from build123d import *
from OCP.BRepFilletAPI import BRepFilletAPI_MakeChamfer

# Parameters (mm, degrees)
SKETCH1_W           = 50
SKETCH1_H           = 40
BODY_DEPTH          = 12
FILLETBODY_R        = 3
SKETCH3_R           = 3.75
BOLT_EXTRUDE_DEPTH  = 1
BOLT_DEPTH          = 10
BOLT_DEPTH_BACK     = 16
SKETCH4_R           = 1.5
SKETCH41_R          = 1.575
CHANNEL1_DEPTH      = 57
SKETCH42_R          = 2.575
INLET_DEPTH         = 5
OUTLET_START        = -5
SKETCH43_R          = 2.575
OUTLET_DEPTH        = 5
SKETCH44_R          = 15
WINDOW_DEPTH        = 5.5
SKETCH45_W          = 16
SKETCH45_H          = 10
FLOWCH_DEPTH        = 5.575
SKETCH46_W          = 10
SKETCH46_H          = 10
WINDOW_HOLE_DEPTH   = 16
SKETCH49_R          = 1.5
FIXHOLES_DEPTH      = 2
GASKET_DEPTH        = 1
CHAMFER_FLOW_SIZE   = 0.5
CHAMFER_FLOW_SIZE_2 = 3


with BuildPart() as part:
    # Sketch1 → Body (new body)
    with BuildSketch(Plane(origin=(0, 0, 0), x_dir=(1, 0, 0), z_dir=(0, 1, 0))):
        Rectangle(SKETCH1_W, SKETCH1_H)
    extrude(amount=BODY_DEPTH)

    # FilletBody
    filletbody_edges = [part.edges().sort_by_distance(p)[0] for p in [
        (-25, 6, -20),
        (25, 6, -20),
        (25, 6, 20),
        (-25, 6, 20),
    ]]
    fillet(filletbody_edges, radius=FILLETBODY_R)

    # Sketch3 → Bolt extrude (add)
    with BuildSketch(Plane(origin=(0, 12, 0), x_dir=(1, 0, 0), z_dir=(0, 1, 0))):
        with Locations(Location((-17.5, 12.5, 0), (0, 0, 270))):
            Circle(SKETCH3_R)
        with Locations(Location((17.5, 12.5, 0), (0, 0, 90))):
            Circle(SKETCH3_R)
        with Locations(Location((17.5, -12.5, 0), (0, 0, 270))):
            Circle(SKETCH3_R)
        with Locations(Location((-17.5, -12.5, 0), (0, 0, 90))):
            Circle(SKETCH3_R)
    extrude(amount=BOLT_EXTRUDE_DEPTH)

    # Sketch4 → Bolt (cut, two sides: drawn at the far end of the back side and taken through both)
    with BuildSketch(Plane(origin=(0, 13, 0), x_dir=(1, 0, 0), z_dir=(0, 1, 0)).offset(-BOLT_DEPTH_BACK)):
        with Locations(Location((-17.5, 12.5, 0), (0, 0, 270))):
            Circle(SKETCH4_R)
        with Locations(Location((17.5, 12.5, 0), (0, 0, 90))):
            Circle(SKETCH4_R)
        with Locations(Location((17.5, -12.5, 0), (0, 0, 270))):
            Circle(SKETCH4_R)
        with Locations(Location((-17.5, -12.5, 0), (0, 0, 90))):
            Circle(SKETCH4_R)
    extrude(amount=BOLT_DEPTH + BOLT_DEPTH_BACK, mode=Mode.SUBTRACT)

    # Sketch41 → Channel1 (cut)
    with BuildSketch(Plane.ZY.offset(25)):
        with Locations((0, 4)):
            Circle(SKETCH41_R)
    extrude(amount=-CHANNEL1_DEPTH, mode=Mode.SUBTRACT)

    # Sketch42 → Inlet (cut)
    with BuildSketch(Plane.ZY.offset(25)):
        with Locations((0, 4)):
            Circle(SKETCH42_R)
    extrude(amount=-INLET_DEPTH, mode=Mode.SUBTRACT)

    # Sketch43 → Outlet (cut)
    with BuildSketch(Plane(origin=(25, 0, 0), x_dir=(0, 0, -1), z_dir=(1, 0, 0)).offset(OUTLET_START)):
        with Locations(Location((0, 4, 0), (0, 0, 180))):
            Circle(SKETCH43_R)
    extrude(amount=OUTLET_DEPTH, mode=Mode.SUBTRACT)

    # Sketch44 → Window (cut)
    with BuildSketch(Plane(origin=(0, 12, 0), x_dir=(1, 0, 0), z_dir=(0, 1, 0))):
        with Locations(Location((0, 0, 0), (0, 0, 270))):
            Circle(SKETCH44_R)
    extrude(amount=-WINDOW_DEPTH, mode=Mode.SUBTRACT)

    # Sketch45 → FlowCh (cut)
    with BuildSketch(Plane.XZ):
        Rectangle(SKETCH45_W, SKETCH45_H)
    extrude(amount=-FLOWCH_DEPTH, mode=Mode.SUBTRACT)

    # Sketch46 → Window_hole (cut)
    with BuildSketch(Plane(origin=(0, 6.5, 0), x_dir=(1, 0, 0), z_dir=(0, 1, 0))):
        Rectangle(SKETCH46_W, SKETCH46_H)
    extrude(amount=-WINDOW_HOLE_DEPTH, mode=Mode.SUBTRACT)

    # Sketch49 → FixHoles (cut)
    with BuildSketch(Plane(origin=(0, 6.5, 0), x_dir=(1, 0, 0), z_dir=(0, 1, 0))):
        with Locations(Location((0, 11, 0), (0, 0, 270))):
            Circle(SKETCH49_R)
        with Locations(Location((0, -11, 0), (0, 0, 270))):
            Circle(SKETCH49_R)
    extrude(amount=-FIXHOLES_DEPTH, mode=Mode.SUBTRACT)

    # Sketch50 → Gasket (cut)
    with BuildSketch(Plane.XZ):
        with BuildLine():
            ThreePointArc((8, 11), (12.242640687, 9.242640687), (14, 5))
            Line((14, 5), (14, -5))
            ThreePointArc((14, -5), (12.242640687, -9.242640687), (8, -11))
            Line((8, -11), (-8, -11))
            ThreePointArc((-8, -11), (-12.242640687, -9.242640687), (-14, -5))
            Line((-14, -5), (-14, 5))
            ThreePointArc((-14, 5), (-12.242640687, 9.242640687), (-8, 11))
            Line((-8, 11), (8, 11))
        make_face()
        with BuildLine():
            Line((-8, -7), (8, -7))
            ThreePointArc((8, -7), (9.414213562, -6.414213562), (10, -5))
            Line((10, -5), (10, 5))
            ThreePointArc((10, 5), (9.414213562, 6.414213562), (8, 7))
            Line((8, 7), (-8, 7))
            ThreePointArc((-8, 7), (-9.414213562, 6.414213562), (-10, 5))
            Line((-10, 5), (-10, -5))
            ThreePointArc((-10, -5), (-9.414213562, -6.414213562), (-8, -7))
        make_face(mode=Mode.SUBTRACT)
    extrude(amount=-GASKET_DEPTH, mode=Mode.SUBTRACT)

    # Chamfer_flow
    chamfer_flow_edges_1 = [part.edges().sort_by_distance(p)[0] for p in [
        (5, 5.575, 0),
    ]]
    chamfer_flow_side_1 = [part.faces().sort_by_distance(p)[0] for p in [
        (5, 5.585, 0),
    ]]
    chamfer_flow_edges_2 = [part.edges().sort_by_distance(p)[0] for p in [
        (-5, 5.575, 0),
    ]]
    chamfer_flow_side_2 = [part.faces().sort_by_distance(p)[0] for p in [
        (-5, 5.585, 0),
    ]]
    chamfer_flow = BRepFilletAPI_MakeChamfer(part.part.solid().wrapped)
    for e in chamfer_flow_edges_1:
        chamfer_flow.Add(CHAMFER_FLOW_SIZE - 0.0001, CHAMFER_FLOW_SIZE_2 - 0.0001, e.wrapped, chamfer_flow_side_1[0].wrapped)
    for e in chamfer_flow_edges_2:
        chamfer_flow.Add(CHAMFER_FLOW_SIZE - 0.0001, CHAMFER_FLOW_SIZE_2 - 0.0001, e.wrapped, chamfer_flow_side_2[0].wrapped)
    add(Compound.cast(chamfer_flow.Shape()), mode=Mode.REPLACE)  # a hair under: the kernel refuses the full size


solid = part.part
Can you work these out from the model? Positions are in its coordinate system, mm. A direction names the side the tool comes from. Give positions to 0.01 mm unless a question says otherwise; leave off trailing zeros. Loops run counter-clockwise (first coordinate to the right, second up) from the corner with the lowest first, then second, coordinate; pieces in that order, holes last. Notation, with made-up numbers: M -19.75,-15.5 L -5.75,-15.5 A29 ccw -5.75,21.5 Z; hole C 51.5,66.5 d11. An arc over 180 degrees is marked long. One line per item, written item: value. Start each with the question number.
1) On a 3-axis mill with a long thin cutter (end or side, diameter ignored), from which of +Z, -Z, +X, -X, +Y, -Y can I reach the whole of each face in a straight line? I mean faces 4 (the face through (22.465, 6.514, -0.558)), 5 (the face through (13.84, 12.49, 11.69)), 6 (the face through (-0.1, 0.5, -7)). Say none if no direction works.
2) If we section it at B-B, the plane y = 9: Write out the boundary of the cut face in (x, z), and give its area (3 significant figures).
3) Thinking about a two-plate mould opening in X: for faces 1 (the face through (13.92, 5.56, -0.21)), 2 (the face through (6.52, 5.82, -0.07)), 3 (the face through (24.14, 6.08, -19.1)), which applies, +X half, -X half, draft (parallel to the pull), parting line (faces both ways), or undercut?
4) If we section it at C-C, the plane x = -3: Write out the boundary of the cut face in (y, z), and give its area (3 significant figures).
5) I'm going to push flat-ended pins straight in: pin 1 (4 mm diameter, centred on y = 4, z = 0, fed in from +X); pin 2 (24 mm diameter, centred on x = -1, z = 4, fed in from +Y); pin 3 (1.5 mm diameter, centred on y = 5, z = 0.5, fed in from -X); pin 4 (5 mm diameter, centred on x = 2, z = 1.5, fed in from -Y). Where does each tip first touch, or does it pass through?
6) If I drill on line 1 (Y direction, x = 16, z = 0) (3 decimals); line 2 (X direction, y = 7.95, z = 0); line 3 (Z direction, x = 19.5, y = 4) (3 decimals), over which ranges is the centre line in solid material (lowest first)? Write a range as [from, to].
7) If we section it at D-D, the plane x = 7: Write out the boundary of the cut face in (y, z), and give its area (3 significant figures).
8) If we section it at A-A, the plane x = -17.5: Write out the boundary of the cut face in (y, z) (3 decimals), and give its area (3 significant figures).
Completed:
1. face 4: +X
1. face 5: +Y
1. face 6: -Y
2. outline: M -25,-17 A3 ccw -22,-20 L 22,-20 A3 ccw 25,-17 L 25,17 A3 ccw 22,20 L -22,20 A3 ccw -25,17 Z; hole C -17.5,-12.5 d3; hole C -17.5,12.5 d3; hole C 0,0 d30; hole C 17.5,-12.5 d3; hole C 17.5,12.5 d3
2. area: 1,260 mm^2
3. face 1: draft
3. face 2: undercut
3. face 3: +X half
4. outline: M 0,-20 L 12,-20 L 12,-14.7 L 6.5,-14.7 L 6.5,-5 L 0,-5 L 0,-7 L 1,-7 L 1,-11 L 0,-11 Z; M 0,5 L 6.5,5 L 6.5,14.7 L 12,14.7 L 12,20 L 0,20 L 0,11 L 1,11 L 1,7 L 0,7 Z
4. area: 245 mm^2
5. pin 1: stops at x = 20
5. pin 2: stops at y = 12
5. pin 3: stops at x = -20
5. pin 4: passes through
6. line 1: y = [0, 2.425], [5.575, 12]
6. line 2: x = [-25, -15], [15, 25]
6. line 3: z = [-20, -1.575], [1.575, 20]
7. outline: M 0,-20 L 12,-20 L 12,-13.27 L 6.5,-13.27 L 6.5,13.27 L 12,13.27 L 12,20 L 0,20 L 0,11 L 1,11 L 1,7 L 0,7 L 0,5 L 5.74,5 L 5.74,-5 L 0,-5 L 0,-7 L 1,-7 L 1,-11 L 0,-11 Z
7. area: 269 mm^2
8. outline: M 0,-20 L 12,-20 L 12,-16.25 L 13,-16.25 L 13,-14 L 0,-14 Z; M 0,-11 L 13,-11 L 13,-8.75 L 12,-8.75 L 12,8.75 L 13,8.75 L 13,11 L 0,11 Z; M 0,14 L 13,14 L 13,16.25 L 12,16.25 L 12,20 L 0,20 Z; hole C 4,0 d3.15
8. area: 409 mm^2
